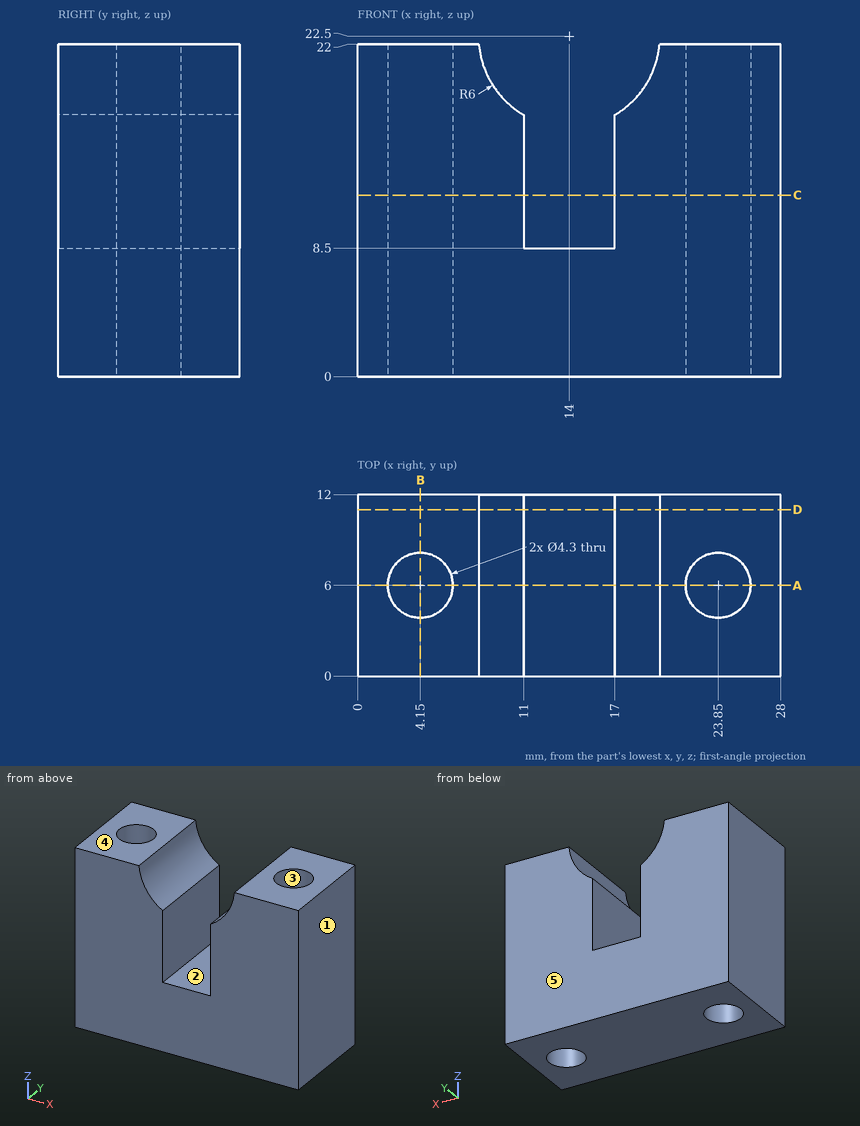
The drawing under review shows one solid part. Ordinate dimensions are in mm from its lowest x, y, z. A direction names the side the tool comes from. Round coordinates to 2 decimals unless told otherwise and drop trailing zeros. Loops run counter-clockwise (first coordinate to the right, second up) from the corner with the lowest first, then second, coordinate; pieces in that order, holes last. Notation, with made-up numbers: (75, 83.25) - (117, 83.25) arc R14 ccw to (117, 96.25) - close; hole circle Ø11 at (10, -21). An arc over 180 degrees is marked (long way). Put each result on its own line as item: value. Start each with the question number.
1. Consider section D-D on y = 11. State the section outline as (x, z) points, plus the area to 3 significant figures.
2. Mouldability with a two-part tool opening along Y and no side actions: class the marked faces 3, 4 and 5 as +Y half, -Y half, draft (parallel to the pull), parting line (faces both ways), or undercut.
3. For probe 1 along X at (y, z) = (6, 6.5); probe 2 along X at (y, z) = (6, 9.75); probe 3 along Y at (x, z) = (23.85, 12.5), list the stretches that pass through material, from the lowest coordinate up. Write a range as [from, to].
4. Insertion check: P1, Ø5, axis at x = 13, y = 8.5, coming from the +Z side. The pin has a flat end and moves straight along its axis. Give the tip position at first contact, or say it passes through.
5. Consider section B-B on x = 4.15. State the section outline as (y, z) points.
6. Consider section C-C on z = 12. State the section outline as (x, y) points.
7. For the marked faces 1 and 2, list the 3-axis set-ups (+Z, -Z, +X, -X, +Y, -Y) from which the entire face can be reached by the end or side of a thin tool; tool diameter is ignored.
8. Consider section A-A on y = 6. State the section outline as (x, z) points.
Result sheet:
1. outline: (0, 0) - (28, 0) - (28, 22) - (19.98, 22) arc R6 cw to (17, 17.3) - (17, 8.5) - (11, 8.5) - (11, 17.3) arc R6 cw to (8.02, 22) - (0, 22) - close
1. area: 516 mm^2
2. face 3: undercut
2. face 4: draft
2. face 5: +Y half
3. probe 1: [0, 2], [6.3, 21.7], [26, 28]
3. probe 2: [0, 2], [6.3, 11], [17, 21.7], [26, 28]
3. probe 3: [0, 3.85], [8.15, 12]
4. P1: z = 17.63
5. outline: (0, 0) - (3.85, 0) - (3.85, 22) - (0, 22) - close; (8.15, 0) - (12, 0) - (12, 22) - (8.15, 22) - close
6. outline: (0, 0) - (11, 0) - (11, 12) - (0, 12) - close; (17, 0) - (28, 0) - (28, 12) - (17, 12) - close; hole circle Ø4.3 at (4.15, 6); hole circle Ø4.3 at (23.85, 6)
7. face 1: +Z, -Z, +X, +Y, -Y
7. face 2: +Z, +Y, -Y
8. outline: (0, 0) - (2, 0) - (2, 22) - (0, 22) - close; (6.3, 0) - (21.7, 0) - (21.7, 22) - (19.98, 22) arc R6 cw to (17, 17.3) - (17, 8.5) - (11, 8.5) - (11, 17.3) arc R6 cw to (8.02, 22) - (6.3, 22) - close; (26, 0) - (28, 0) - (28, 22) - (26, 22) - close
